Part print with two shaded views. Sizes in mm from the minimum x, y, z corner. A direction names the side the tool comes from. Give positions to 0.01 mm unless a question says otherwise; leave off trailing zeros. Write each loop counter-clockwise with the first axis right and the second up, starting at its lowest first coordinate (ties: lowest second). Pieces come first, ordered by that corner, then holes.
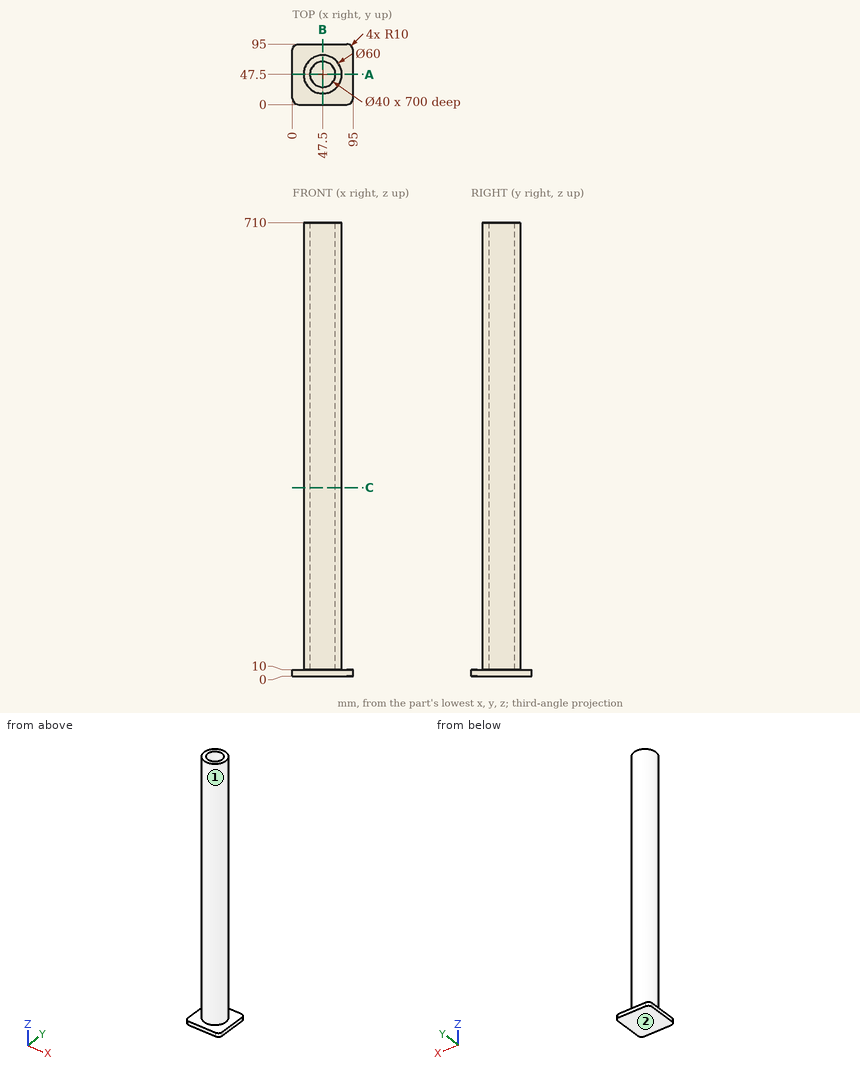
1) Drill centre lines: L1, parallel to Y at x = 47, z = 491; L2, parallel to X at y = 49, z = 585. Where is each one in solid material? Low to high.
Check result:
L1: y = 17.5 to 27.51, 67.49 to 77.5
L2: x = 17.54 to 27.56, 67.44 to 77.46
2) Flat gauge pins, fed straight in: P1, Ø1, axis at x = 62.5, y = 36.5, coming from the +Z side; P2, Ø1.5, axis at x = 70.5, y = 50.5, coming from the -Z side; P3, Ø3, axis at x = 46.5, z = 231, coming from the +Y side; P4, Ø8, axis at y = 64, z = 334.5, coming from the -X side. Where does each tip first touch, or does it go through?
Check result:
P1: stops at z = 10
P2: stops at z = 0
P3: stops at y = 77.5
P4: stops at x = 20.23
3) Saw through at A-A (y = 47.5). Write the cut outline in (x, z).
Check result:
outline: (0, 0) - (95, 0) - (95, 10) - (77.5, 10) - (77.5, 710) - (67.5, 710) - (67.5, 10) - (27.5, 10) - (27.5, 710) - (17.5, 710) - (17.5, 10) - (0, 10) - close
4) 3-axis set-ups, long thin cutter, end or side, ignore diameter. For the marked faces 1 and 2: which of +Z, -Z, +X, -X, +Y, -Y reach the whole face in a straight line?
Check result:
face 1: +Z
face 2: -Z, +X, -X, +Y, -Y
5) Saw through at C-C (z = 295). Write the cut outline in (x, y), and give its area (3 significant figures).
Check result:
outline: circle Ø60 at (47.5, 47.5); hole circle Ø40 at (47.5, 47.5)
area: 1,570 mm2
